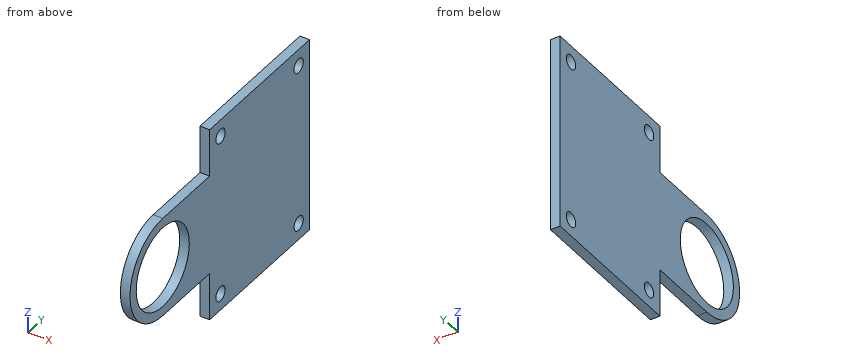
from build123d import *

# Parameters (mm, degrees)
SKETCH_1_R      = 8.5
SKETCH_1_R_2    = 1.5
EXTRUDE_1_DEPTH = 2


with BuildPart() as part:
    # 草图1 → 凸台-拉伸1 (new body)
    with BuildSketch(Plane(origin=(0, 0, 0), x_dir=(0, 0, -1), z_dir=(1, 0, 0))):
        with BuildLine():
            Line((-10.5, 0), (-10.5, 15))
            Line((-10.5, 15), (-20.5, 15))
            Line((-20.5, 15), (-20.5, 47))
            Line((-20.5, 47), (20.5, 47))
            Line((20.5, 47), (20.5, 15))
            Line((20.5, 15), (10.5, 15))
            Line((10.5, 15), (10.5, 0))
            ThreePointArc((10.5, 0), (0, -10.5), (-10.5, 0))
        make_face()
        Circle(SKETCH_1_R, mode=Mode.SUBTRACT)
        with Locations((-17, 43.5)):
            Circle(SKETCH_1_R_2, mode=Mode.SUBTRACT)
        with Locations((17, 43.5)):
            Circle(SKETCH_1_R_2, mode=Mode.SUBTRACT)
        with Locations((-17, 18.5)):
            Circle(SKETCH_1_R_2, mode=Mode.SUBTRACT)
        with Locations((17, 18.5)):
            Circle(SKETCH_1_R_2, mode=Mode.SUBTRACT)
    extrude(amount=EXTRUDE_1_DEPTH)


solid = part.part
The model under review builds one solid part; all positions refer to its coordinate system, in mm. Give positions to 0.01 mm unless a question says otherwise; leave off trailing zeros. Order: outer loops, then holes, each group sorted by start corner. A loop starts at its lowest first (then second) coordinate and runs counter-clockwise, first axis right, second up. Notation, with made-up numbers: M 87,64.25 L 137,64.25 A34 cw 137,103.25 Z; hole C 29,55 d3. An arc over 180 degrees is marked long. Answer in a Markdown table with one row per item. Add a question column.
1. To check wall thickness, follow line 1 along Y through (x, z) = (0.9, -17); line 2 along Y through (x, z) = (1.25, -14); line 3 along Y through (x, z) = (1.25, 0). State the ranges of each line that lie inside material, in increasing order.
2. Add section D-D on y = -2. State the section outline as (x, z) points, plus the area to 3 significant figures.
3. Add section C-C on x = 1.65. State the section outline as (y, z) points, plus the area to 3 significant figures.
4. Add section B-B on z = 0. State the section outline as (x, y) points.
5. For pin 1 Ø1 at (x, y) = (1, 4.5) entering from -Z; pin 2 Ø0.6 at (x, z) = (1, -17) entering from -Y, all flat-tipped, find the tip position at first contact; note any pin that passes through.
6. Add section A-A on y = 43.5. State the section outline as (x, z) points.
The answers:
| question | item | result |
|---|---|---|
| 1 | line 1 | 15 to 17, 20 to 42, 45 to 47 |
| 1 | line 2 | 15 to 47 |
| 1 | line 3 | -10.5 to -8.5, 8.5 to 47 |
| 2 | outline | M 0,-10.31 L 2,-10.31 L 2,-8.26 L 0,-8.26 Z; M 0,8.26 L 2,8.26 L 2,10.31 L 0,10.31 Z |
| 2 | area | 8.19 mm2 |
| 3 | outline | M 0,-10.5 L 15,-10.5 L 15,-20.5 L 47,-20.5 L 47,20.5 L 15,20.5 L 15,10.5 L 0,10.5 A10.5 ccw Z; hole C 0,0 d17; hole C 18.5,-17 d3; hole C 18.5,17 d3; hole C 43.5,-17 d3; hole C 43.5,17 d3 |
| 3 | area | 1,540 mm2 |
| 4 | outline | M 0,-10.5 L 2,-10.5 L 2,-8.5 L 0,-8.5 Z; M 0,8.5 L 2,8.5 L 2,47 L 0,47 Z |
| 5 | pin 1 | z = -10.5 |
| 5 | pin 2 | y = 15 |
| 6 | outline | M 0,-20.5 L 2,-20.5 L 2,-18.5 L 0,-18.5 Z; M 0,-15.5 L 2,-15.5 L 2,15.5 L 0,15.5 Z; M 0,18.5 L 2,18.5 L 2,20.5 L 0,20.5 Z |
